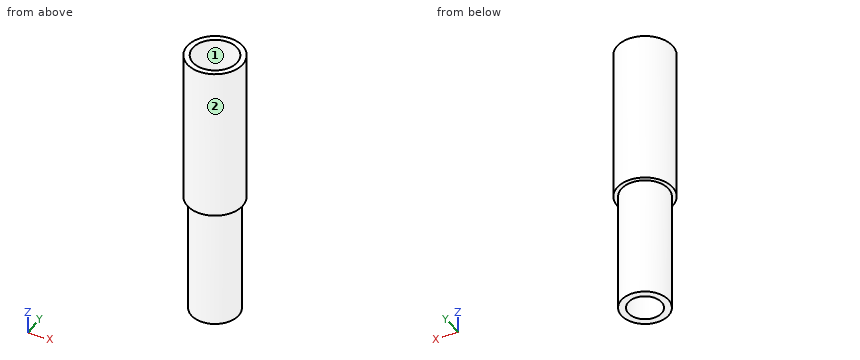
from build123d import *

# Parameters (mm, degrees)
SKETCH_R        = 5
PAD_DEPTH       = 50
SKETCH001_R     = 2
POCKET_DEPTH    = 50.001
SKETCH002_R     = 4
POCKET001_DEPTH = 25
SKETCH003_R     = 3
POCKET002_DEPTH = 20
SKETCH004_R     = 5
SKETCH004_R_2   = 4.25
POCKET003_DEPTH = 22


with BuildPart() as part:
    # Sketch → Pad (new body)
    with BuildSketch(Plane.XY):
        Circle(SKETCH_R)
    extrude(amount=PAD_DEPTH)

    # Sketch001 → Pocket (cut, through all)
    with BuildSketch(Plane.XY.offset(50)):
        Circle(SKETCH001_R)
    extrude(amount=-POCKET_DEPTH, mode=Mode.SUBTRACT)

    # Sketch002 → Pocket001 (cut)
    with BuildSketch(Plane.XY.offset(50)):
        Circle(SKETCH002_R)
    extrude(amount=-POCKET001_DEPTH, mode=Mode.SUBTRACT)

    # Sketch003 → Pocket002 (cut)
    with BuildSketch(Plane(origin=(0, 0, 0), x_dir=(1, 0, 0), z_dir=(0, 0, -1))):
        Circle(SKETCH003_R)
    extrude(amount=-POCKET002_DEPTH, mode=Mode.SUBTRACT)

    # Sketch004 → Pocket003 (cut)
    with BuildSketch(Plane(origin=(0, 0, 0), x_dir=(1, 0, 0), z_dir=(0, 0, -1))):
        Circle(SKETCH004_R)
        Circle(SKETCH004_R_2, mode=Mode.SUBTRACT)
    extrude(amount=-POCKET003_DEPTH, mode=Mode.SUBTRACT)


solid = part.part
The model under review builds one solid part; all positions refer to its coordinate system, in mm. Face numbers are marked on the shaded views. Give positions to 0.01 mm unless a question says otherwise; leave off trailing zeros. Loops run counter-clockwise (first coordinate to the right, second up) from the corner with the lowest first, then second, coordinate; pieces in that order, holes last. Notation, with made-up numbers: (69.25, 68.5) -> (117.25, 68.5) arc R33 cw to (117.25, 100.5) -> close; hole circle Ø10 at (-31, -34.75). An arc over 180 degrees is marked (long way). Answer as a JSON object with one key per item and string values. Group by question number.
Q1. Take a section at A-A (x = 0). Write out the cut boundary in (y, z), plus the area to 3 significant figures.
Q2. Draft analysis for pull direction Y (two halves, no side actions). For the marked faces 1 and 2, state which applies: pulls with the +Y half, pulls with the -Y half, needs draft (parallel to the pull), parting line crosses it, or undercut.
Q3. Take a section at B-B (y = -1.5). Write out the cut boundary in (x, z).
Q4. Take a section at C-C (z = 19). Write out the cut boundary in (x, y), plus the area to 3 significant figures.
Q5. Wall thickness on line 1 along Y through (x, z) = (0, 9); line 2 along Y through (x, z) = (0, 21.4): over which ranges is each line inside the solid? List them lowest first.
Q6. Take a section at D-D (z = 41.5). Write out the cut boundary in (x, y).
Q7. Insertion check: pin 1 (1 mm diameter, centred on x = 1, z = 41.5, fed in from +Y); pin 2 (4 mm diameter, centred on x = 4, z = 42.5, fed in from +Y); pin 3 (6 mm diameter, centred on y = -3.5, z = 40.5, fed in from +X). Each pin has a flat end and moves straight along its axis. Give the tip position at first contact, or say it passes through.
Answer below:
{
 "1": {"outline": "(-5, 22) -> (-4.25, 22) -> (-4.25, 0) -> (-3, 0) -> (-3, 20) -> (-2, 20) -> (-2, 25) -> (-4, 25) -> (-4, 50) -> (-5, 50) -> close; (2, 20) -> (3, 20) -> (3, 0) -> (4.25, 0) -> (4.25, 22) -> (5, 22) -> (5, 50) -> (4, 50) -> (4, 25) -> (2, 25) -> close", "area": "127 mm2"},
 "2": {"face 1": "undercut", "face 2": "parting line crosses it"},
 "3": {"outline": "(-4.77, 22) -> (-3.98, 22) -> (-3.98, 0) -> (-2.6, 0) -> (-2.6, 20) -> (-1.32, 20) -> (-1.32, 25) -> (-3.71, 25) -> (-3.71, 50) -> (-4.77, 50) -> close; (1.32, 20) -> (2.6, 20) -> (2.6, 0) -> (3.98, 0) -> (3.98, 22) -> (4.77, 22) -> (4.77, 50) -> (3.71, 50) -> (3.71, 25) -> (1.32, 25) -> close"},
 "4": {"outline": "circle Ø8.5 at (0, 0); hole circle Ø6 at (0, 0)", "area": "28.5 mm2"},
 "5": {"line 1": "y = -4.25 to -3, 3 to 4.25", "line 2": "y = -4.25 to -2, 2 to 4.25"},
 "6": {"outline": "circle Ø10 at (0, 0); hole circle Ø8 at (0, 0)"},
 "7": {"pin 1": "stops at y = 4.97", "pin 2": "stops at y = 4.58", "pin 3": "stops at x = 4.97"}
}
